Verification items for the finished model (mm, model axes). A direction names the side the tool comes from. Coordinates: 2 decimals unless noted, no trailing zeros. Write each loop counter-clockwise with the first axis right and the second up, starting at its lowest first coordinate (ties: lowest second). Pieces come first, ordered by that corner, then holes. Notation, with made-up numbers: (2.25, 16) -> (38.25, 16) arc R26 ccw to (38.25, 42) -> close; hole circle Ø6 at (47.5, 3). An arc over 180 degrees is marked (long way). Answer in a Markdown table with one row per item.
```python
from build123d import *

# Parameters (mm, degrees)
F0_W          = 15
F0_H          = 50
F1_DEPTH      = 142.5
F1_DEPTH_BACK = 142.5
F2_W          = 15
F2_H          = 50
F3_DEPTH      = 17.5
F4_R          = 2


# Not quite as in the source:
# - a pattern or mirror of a feature is missing from the dataset's text; its kind, count and spacing are read off the source's solid


with BuildPart() as f1:
    # F0 (on Front) → F1 (new body, two sides)
    with BuildSketch(Plane.XZ) as f1_sk:
        Rectangle(F0_W, F0_H)
    extrude(amount=F1_DEPTH)
    extrude(f1_sk.sketch, amount=-F1_DEPTH_BACK)

    # F2 (on face) → F3 (cut)
    with BuildSketch(Plane.XZ.offset(142.5)):
        Rectangle(F2_W, F2_H)
        with BuildLine():
            ThreePointArc((5, -15), (0, -20), (-5, -15))
            Line((-5, -15), (-5, 15))
            ThreePointArc((-5, 15), (0, 20), (5, 15))
            Line((5, 15), (5, -15))
        make_face(mode=Mode.SUBTRACT)
    f3 = extrude(amount=-F3_DEPTH, mode=Mode.SUBTRACT)

    # F3_copies: F3 across plane
    add(f3.mirror(Plane.ZX), mode=Mode.SUBTRACT)

    # F4
    f4_edges = [f1.edges().sort_by_distance(p)[0] for p in [
        (7.5, 0, -25),
        (-7.5, 0, -25),
    ]]
    fillet(f4_edges, radius=F4_R)


solid = f1.part
```
1. Sectioned sample at A-A, the plane x = 0. Record the cut outline in (y, z), and give its area (3 significant figures).
Findings below:
| item | result |
|---|---|
| outline | (-142.5, -20) -> (-125, -20) -> (-125, -25) -> (125, -25) -> (125, -20) -> (142.5, -20) -> (142.5, 20) -> (125, 20) -> (125, 25) -> (-125, 25) -> (-125, 20) -> (-142.5, 20) -> close |
| area | 13,900 mm² |
2. Access from +Z, -Z, +X, -X, +Y, -Y to the whole of each face (thin tool, end or side, straight path). Record for faces 1 (the face through (-5, 134, 0)), 2 (the face through (0, -134, -20)), 3 (the face through (-7, -125, 0)), 4 (the face through (5, 134, 0)), 5 (the face through (-5, -134, 0)).
Findings below:
| item | result |
|---|---|
| face 1 | +Z, -Z, -X, +Y |
| face 2 | -Z, -Y |
| face 3 | -Y |
| face 4 | +Z, -Z, +X, +Y |
| face 5 | +Z, -Z, -X, -Y |
3. Material ranges on probe 1 along X at (y, z) = (128.5, -8); probe 2 along Y at (x, z) = (5, 19); probe 3 along Z at (x, y) = (6.75, -29), recorded low to high. Write a range as from..to.
Findings below:
| item | result |
|---|---|
| probe 1 | x = -5..5 |
| probe 2 | y = -125..125 |
| probe 3 | z = -24.56..25 |
4. Go/stop test with flat-tipped pins: pin 1 (5 mm diameter, centred on y = -138, z = 3, fed in from +X); pin 2 (9 mm diameter, centred on y = -131, z = 6, fed in from -X). Record where each tip stops, or that it passes through.
Findings below:
| item | result |
|---|---|
| pin 1 | stops at x = 5 |
| pin 2 | stops at x = -5 |
